```python
from build123d import *

# Parameters (mm, degrees)
SKETCH1_W           = 400.05
SKETCH1_H           = 279.4
SKETCH1_R           = 3.175
SKETCH1_W_2         = 71.12
SKETCH1_H_2         = 71.12
BOSS_EXTRUDE1_DEPTH = 3.175


with BuildPart() as part:
    # Sketch1 → Boss-Extrude1 (new body)
    with BuildSketch(Plane.XY):
        Rectangle(SKETCH1_W, SKETCH1_H)
        with Locations((-85.725, 88.9)):
            Circle(SKETCH1_R, mode=Mode.SUBTRACT)
        with Locations((-121.285, 88.9)):
            Circle(SKETCH1_R, mode=Mode.SUBTRACT)
        with Locations((-50.165, 88.9)):
            Circle(SKETCH1_R, mode=Mode.SUBTRACT)
        with Locations((-50.165, 101.6)):
            Circle(SKETCH1_R, mode=Mode.SUBTRACT)
        with Locations((-85.725, 101.6)):
            Circle(SKETCH1_R, mode=Mode.SUBTRACT)
        with Locations((-121.285, 101.6)):
            Circle(SKETCH1_R, mode=Mode.SUBTRACT)
        with Locations(Location((121.285, 88.9, 0), (0, 0, 180))):
            Circle(SKETCH1_R, mode=Mode.SUBTRACT)
        with Locations(Location((85.725, 88.9, 0), (0, 0, 180))):
            Circle(SKETCH1_R, mode=Mode.SUBTRACT)
        with Locations(Location((50.165, 88.9, 0), (0, 0, 180))):
            Circle(SKETCH1_R, mode=Mode.SUBTRACT)
        with Locations(Location((50.165, 101.6, 0), (0, 0, 180))):
            Circle(SKETCH1_R, mode=Mode.SUBTRACT)
        with Locations(Location((85.725, 101.6, 0), (0, 0, 180))):
            Circle(SKETCH1_R, mode=Mode.SUBTRACT)
        with Locations(Location((121.285, 101.6, 0), (0, 0, 180))):
            Circle(SKETCH1_R, mode=Mode.SUBTRACT)
        with Locations((-85.725, 38.1)):
            Rectangle(SKETCH1_W_2, SKETCH1_H_2, mode=Mode.SUBTRACT)
        with Locations((85.725, 38.1)):
            Rectangle(SKETCH1_W_2, SKETCH1_H_2, mode=Mode.SUBTRACT)
    extrude(amount=BOSS_EXTRUDE1_DEPTH)


solid = part.part
```
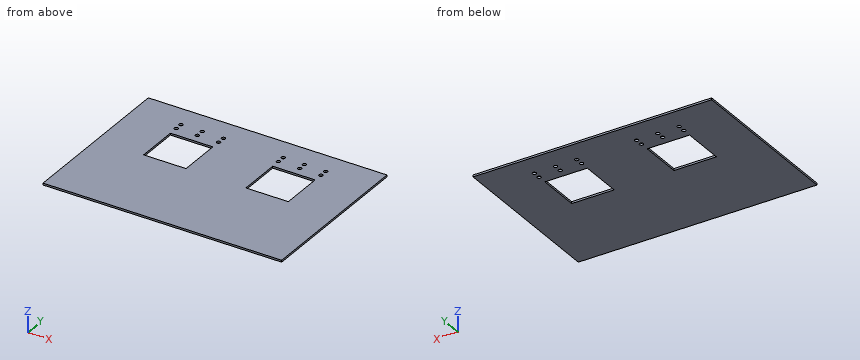
Can you work these out from the model? Positions are in its coordinate system, mm. Give positions to 0.01 mm unless a question says otherwise; leave off trailing zeros. Write each loop counter-clockwise with the first axis right and the second up, starting at its lowest first coordinate (ties: lowest second). Pieces come first, ordered by that corner, then holes. Notation, with made-up numbers: (-6, 57.25) -> (9, 57.25) arc R24 ccw to (9, 76.25) -> close; hole circle Ø9 at (37.25, 27). An arc over 180 degrees is marked (long way). One line per item, written item: value.
Q1. Please list where these lines run through material, in increasing order: line 1 (X direction, y = 33, z = 1.3) (3 decimals); line 2 (Y direction, x = 113, z = 2.3); line 3 (Y direction, x = 51.5, z = 0.25). Write a range as [from, to].
Results found:
line 1: x = [-200.025, -121.285], [-50.165, 50.165], [121.285, 200.025]
line 2: y = [-139.7, 2.54], [73.66, 139.7]
line 3: y = [-139.7, 2.54], [73.66, 86.02], [91.78, 98.72], [104.48, 139.7]
Q2. For P1, Ø5.5, axis at x = 85.725, y = 88.9, coming from the +Z side, with a flat end and sliding along its axis, tell me the tip position at first contact or that it passes through.
Results found:
P1: passes through
Q3. Imagine slicing it at B-B on x = 63.5. Please give me the cut outline in (y, z) (3 decimals), and give its area (3 significant figures).
Results found:
outline: (-139.7, 0) -> (2.54, 0) -> (2.54, 3.175) -> (-139.7, 3.175) -> close; (73.66, 0) -> (139.7, 0) -> (139.7, 3.175) -> (73.66, 3.175) -> close
area: 661 mm^2
Q4. Imagine slicing it at C-C on z = 1.5. Give the number of separate pieces and of enclosed holes in the cut face, and give its area (3 significant figures).
Results found:
separate pieces: 1
enclosed holes: 14
area: 101,000 mm^2
Q5. Imagine slicing it at A-A on y = 35. Please give me the cut outline in (x, z) (3 decimals).
Results found:
outline: (-200.025, 0) -> (-121.285, 0) -> (-121.285, 3.175) -> (-200.025, 3.175) -> close; (-50.165, 0) -> (50.165, 0) -> (50.165, 3.175) -> (-50.165, 3.175) -> close; (121.285, 0) -> (200.025, 0) -> (200.025, 3.175) -> (121.285, 3.175) -> close
